```python
from build123d import *

# Parameters (mm, degrees)
F0_W     = 185.9026
F0_H     = 47.5996
F1_DEPTH = 12.7
F2_R     = 2.54
F3_DEPTH = 2.54
F4_R     = 2.54
F5_DEPTH = 2.54
F6_W     = 173.2026
F6_H     = 22.1996
F7_DEPTH = 7.62
F8_W     = 178.2826
F8_H     = 27.2796
F9_DEPTH = 6.35


with BuildPart() as f1:
    # F0 (on Top) → F1 (new body)
    with BuildSketch(Plane.XY):
        Rectangle(F0_W, F0_H)
    extrude(amount=F1_DEPTH)

    # F2 (on face) → F3 (cut)
    with BuildSketch(Plane.YZ.offset(92.9513)):
        with Locations((0, 6.35)):
            Circle(F2_R)
    extrude(amount=-F3_DEPTH, mode=Mode.SUBTRACT)

    # F4 (on face) → F5 (cut)
    with BuildSketch(Plane(origin=(-92.9513, 0, 0), x_dir=(0, -1, 0), z_dir=(-1, 0, 0))):
        with Locations((0, 6.35)):
            Circle(F4_R)
    extrude(amount=-F5_DEPTH, mode=Mode.SUBTRACT)

    # F6 (on face) → F7 (cut)
    with BuildSketch(Plane.XY.offset(12.7)):
        Rectangle(F6_W, F6_H)
    extrude(amount=-F7_DEPTH, mode=Mode.SUBTRACT)

    # F8 (on face) → F9 (cut)
    with BuildSketch(Plane.XY.offset(12.7)):
        Rectangle(F8_W, F8_H)
    extrude(amount=-F9_DEPTH, mode=Mode.SUBTRACT)


solid = f1.part
```
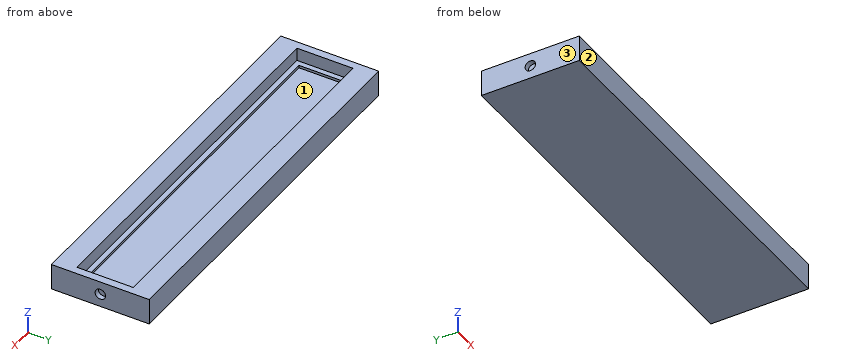
The model under review builds one solid part; all positions refer to its coordinate system, in mm. Face numbers are marked on the shaded views. Round coordinates to 2 decimals unless told otherwise and drop trailing zeros. Write each loop counter-clockwise with the first axis right and the second up, starting at its lowest first coordinate (ties: lowest second). Pieces come first, ordered by that corner, then holes. Notation, with made-up numbers: (24, -18) - (59, -18) arc R31 cw to (59, 8) - close; hole circle Ø7 at (2, -37). An arc over 180 degrees is marked (long way). Use one line per item in the form item = value.
Q1. Insertion check: pin 1 Ø2.5 at (y, z) = (0.5, 5.5) entering from -X; pin 2 Ø1.5 at (y, z) = (-1, 7.5) entering from +X. Each pin has a flat end and moves straight along its axis. Give the tip position at first contact, or say it passes through.
Answer key:
pin_1 = -90.41
pin_2 = 90.41
Q2. Consider section A-A (y = 0). State the section outline as (x, z) points, and give its area (3 significant figures).
Answer key:
outline = (-92.95, 0) - (92.95, 0) - (92.95, 3.81) - (90.41, 3.81) - (90.41, 8.89) - (92.95, 8.89) - (92.95, 12.7) - (89.14, 12.7) - (89.14, 6.35) - (86.6, 6.35) - (86.6, 5.08) - (-86.6, 5.08) - (-86.6, 6.35) - (-89.14, 6.35) - (-89.14, 12.7) - (-92.95, 12.7) - (-92.95, 8.89) - (-90.41, 8.89) - (-90.41, 3.81) - (-92.95, 3.81) - close
area = 983 mm2
Q3. Consider section B-B (x = -61.5). State the section outline as (y, z) points, and give its area (3 significant figures).
Answer key:
outline = (-23.8, 0) - (23.8, 0) - (23.8, 12.7) - (13.64, 12.7) - (13.64, 6.35) - (11.1, 6.35) - (11.1, 5.08) - (-11.1, 5.08) - (-11.1, 6.35) - (-13.64, 6.35) - (-13.64, 12.7) - (-23.8, 12.7) - close
area = 403 mm2
Q4. Draft analysis for pull direction Y (two halves, no side actions). For the marked faces 1, 2 and 3, state which applies: +Y half, -Y half, draft (parallel to the pull), parting line (faces both ways), or undercut.
Answer key:
face_1 = undercut
face_2 = -Y half
face_3 = draft
Q5. For line 1 (Z direction, x = -91.7, y = 0); line 2 (X direction, y = -11.5, z = 11.75); line 3 (Y direction, x = 23.5, z = 6), list the stretches that pass through material, from the lowest coordinate up. Write a range as [from, to].
Answer key:
line_1 = [0, 3.81], [8.89, 12.7]
line_2 = [-92.95, -89.14], [89.14, 92.95]
line_3 = [-23.8, -11.1], [11.1, 23.8]
